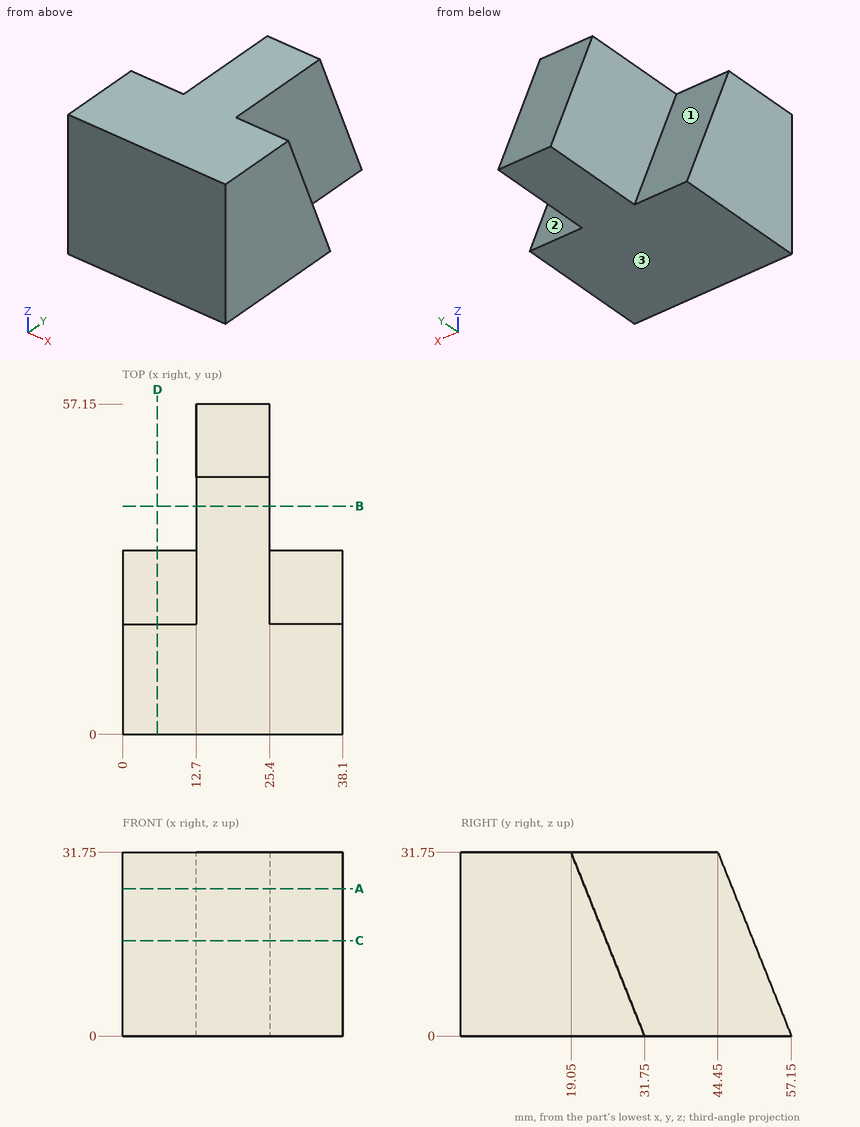
Job drawing, mm, ordinate dimensions from the low corner. One solid piece. A direction names the side the tool comes from. Round coordinates to 2 decimals unless told otherwise and drop trailing zeros. Write each loop counter-clockwise with the first axis right and the second up, starting at its lowest first coordinate (ties: lowest second). Pieces come first, ordered by that corner, then holes. Notation, with made-up numbers: M -38,64 L 10,64 A13 cw 10,85 Z; hole C -34.5,67 d5. An arc over 180 degrees is marked long. Return JSON: item names as keys, results as strings. Group by question number.
(1) Saw through at C-C on z = 16.5. Write the cut outline in (x, y), then the cut area to 3 significant figures.
(2) Pin check, flat tips, straight feed: pin 1 Ø2 at (x, z) = (6, 7.5) entering from +Y; pin 2 Ø2 at (y, z) = (44.5, 7.5) entering from +X; pin 3 Ø10 at (x, z) = (18.5, 23.5) entering from +Y. Stop position of each tip, or through.
(3) Drill centre lines: probe 1 along X at (y, z) = (33, 18.5); probe 2 along Y at (x, z) = (3, 8); probe 3 along Y at (x, z) = (27, 20). Where is each one in solid material? Low to high.
(4) Saw through at A-A on z = 25.5. Write the cut outline in (x, y), then the cut area to 3 significant figures.
(5) Which spindle directions (+Z, -Z, +X, -X, +Y, -Y) get a long thin tool onto all of the face, cutting with end or side? Do the marked faces 1, 2 and 3. Say none if no direction does.
(6) Saw through at D-D on x = 6. Write the cut outline in (y, z), then the cut area to 3 significant figures.
(7) Saw through at B-B on y = 39.5. Write the cut outline in (x, z).
Returned:
{
 "1": {"outline": "M 0,0 L 38.1,0 L 38.1,25.15 L 25.4,25.15 L 25.4,50.55 L 12.7,50.55 L 12.7,25.15 L 0,25.15 Z", "area": "1,280 mm²"},
 "2": {"pin 1": "y = 29.15", "pin 2": "x = 25.4", "pin 3": "y = 49.75"},
 "3": {"probe 1": "12.7 to 25.4", "probe 2": "0 to 28.55", "probe 3": "0 to 23.75"},
 "4": {"outline": "M 0,0 L 38.1,0 L 38.1,21.55 L 25.4,21.55 L 25.4,46.95 L 12.7,46.95 L 12.7,21.55 L 0,21.55 Z", "area": "1,140 mm²"},
 "5": {"face 1": "+Z, -X, +Y", "face 2": "+Z, +X, +Y", "face 3": "-Z, +X, -X, +Y, -Y"},
 "6": {"outline": "M 0,0 L 31.75,0 L 19.05,31.75 L 0,31.75 Z", "area": "806 mm²"},
 "7": {"outline": "M 12.7,0 L 25.4,0 L 25.4,31.75 L 12.7,31.75 Z"}
}
